from build123d import *

# Parameters (mm, degrees)
SKETCH1_R             = 22.225
BOSS_EXTRUDE1_DEPTH   = 50.8
SKETCH2_R             = 22.225
SKETCH2_R_2           = 15.375
CUT_EXTRUDE1_DEPTH    = 30.1625
SKETCH3_R             = 12.7
CUT_EXTRUDE2_DEPTH    = 49.2125
CUT_EXTRUDE3_START    = -17.4625
SKETCH5_R             = 22.225
SKETCH5_R_2           = 15.875
CUT_EXTRUDE3_DEPTH    = 17.4625
SKETCH6_R             = 8.001
SKETCH6_R_2           = 1.70053
MOTORINTERFACFE_DEPTH = 60.737268518


with BuildPart() as part:
    # Sketch1 → Boss-Extrude1 (new body)
    with BuildSketch(Plane(origin=(0, 0, 0), x_dir=(1, 0, 0), z_dir=(0, 1, 0))):
        with Locations(Location((0, 0, 0), (0, 0, 270))):
            Circle(SKETCH1_R)
    extrude(amount=BOSS_EXTRUDE1_DEPTH)

    # Sketch2 → Cut-Extrude1 (cut)
    with BuildSketch(Plane.XZ):
        with Locations(Location((0, 0, 0), (0, 0, 270))):
            Circle(SKETCH2_R)
        with Locations(Location((0, 0, 0), (0, 0, 270))):
            Circle(SKETCH2_R_2, mode=Mode.SUBTRACT)
    extrude(amount=-CUT_EXTRUDE1_DEPTH, mode=Mode.SUBTRACT)

    # Sketch3 → Cut-Extrude2 (cut)
    with BuildSketch(Plane(origin=(0, 50.8, 0), x_dir=(1, 0, 0), z_dir=(0, 1, 0))):
        with Locations(Location((0, 0, 0), (0, 0, 270))):
            Circle(SKETCH3_R)
    extrude(amount=-CUT_EXTRUDE2_DEPTH, mode=Mode.SUBTRACT)

    # Sketch5 → Cut-Extrude3 (cut)
    with BuildSketch(Plane(origin=(0, 50.8, 0), x_dir=(1, 0, 0), z_dir=(0, 1, 0)).offset(CUT_EXTRUDE3_START)):
        with Locations(Location((0, 0, 0), (0, 0, 90))):
            Circle(SKETCH5_R)
        with Locations(Location((0, 0, 0), (0, 0, 270))):
            Circle(SKETCH5_R_2, mode=Mode.SUBTRACT)
    extrude(amount=CUT_EXTRUDE3_DEPTH, mode=Mode.SUBTRACT)

    # Sketch6 → MotorInterfacfe (cut, through all)
    with BuildSketch(Plane.XZ):
        with Locations(Location((0, 0, 0), (0, 0, 270))):
            Circle(SKETCH6_R)
        with Locations(Location((-7.07105367, 7.07105367, 0), (0, 0, 270))):
            Circle(SKETCH6_R_2)
        with Locations(Location((-7.162899066, -6.970031681, 0), (0, 0, 270))):
            Circle(SKETCH6_R_2)
        with Locations(Location((7.158557907, -7.103864696, 0), (0, 0, 270))):
            Circle(SKETCH6_R_2)
        with Locations(Location((7.036006619, 7.187404798, 0), (0, 0, 270))):
            Circle(SKETCH6_R_2)
    extrude(amount=-MOTORINTERFACFE_DEPTH, mode=Mode.SUBTRACT)


solid = part.part
Work out the finished part from the listing and answer in its coordinate system (mm). A direction names the side the tool comes from. Coordinates: 2 decimals unless noted, no trailing zeros. Loops run counter-clockwise (first coordinate to the right, second up) from the corner with the lowest first, then second, coordinate; pieces in that order, holes last. Notation, with made-up numbers: (82.25, 56) -> (95.25, 56) arc R19 cw to (95.25, 74) -> close; hole circle Ø2 at (9.25, 45.5). An arc over 180 degrees is marked (long way). Answer as CSV lines item,"result".
1) Straight lines are drawn through the part: probe 1 along X at (y, z) = (23, 0) (3 decimals); probe 2 along X at (y, z) = (1.1, 0) (3 decimals); probe 3 along Y at (x, z) = (9, 1). For each, find the intervals that lie inside material, in ascending order.
A:
probe 1,"x = -15.375 to -12.7, 12.7 to 15.375"
probe 2,"x = -15.375 to -8.001, 8.001 to 15.375"
probe 3,"y = 0 to 1.59"
2) For faces 1 (the face through (-15, 30.162, 5)), 2 (the face through (-8.3, 1.587, -0.2)), 3 (the face through (2.403, 0.783, -7.632)), determine the directions among +Z, -Z, +X, -X, +Y, -Y from which every point of the face is accessible in a straight line to the end or side of a thin tool.
A:
face 1,"-Y"
face 2,"+Y"
face 3,"+Y, -Y"
3) The part is cut by section D-D (y = 24.5). Give the vertices of the cut face in (x, z) (3 decimals).
A:
outline,"circle Ø30.75 at (0, 0); hole circle Ø25.4 at (0, 0)"
4) The part is cut by section C-C (z = -6.5). Give the vertices of the cut face in (x, y), and give its area (3 significant figures).
A:
outline,"(-21.25, 30.16) -> (-13.93, 30.16) -> (-13.93, 0) -> (-8.8, 0) -> (-8.8, 1.59) -> (-10.91, 1.59) -> (-10.91, 50.8) -> (-14.48, 50.8) -> (-14.48, 33.34) -> (-21.25, 33.34) -> close; (-5.53, 0) -> (-4.67, 0) -> (-4.67, 1.59) -> (-5.53, 1.59) -> close; (4.67, 0) -> (5.57, 0) -> (5.57, 1.59) -> (4.67, 1.59) -> close; (8.75, 0) -> (13.93, 0) -> (13.93, 30.16) -> (21.25, 30.16) -> (21.25, 33.34) -> (14.48, 33.34) -> (14.48, 50.8) -> (10.91, 50.8) -> (10.91, 1.59) -> (8.75, 1.59) -> close"
area,"382 mm²"
5) For a pull along X with two mould halves and no side action, classify faces 4 (the face through (11, 50.8, -7)), 5 (the face through (-8.73, 0.78, 7.44)), 6 (the face through (-15.497, 41.947, -3.441)) as released by +X, released by -X, zero draft, split by the parting line, or undercut.
A:
face 4,"zero draft"
face 5,"undercut"
face 6,"split by the parting line"
6) The part is cut by section B-B (x = 0). Give the vertices of the cut face in (y, z) (1 decimal).
A:
outline,"(0, -15.4) -> (30.2, -15.4) -> (30.2, -22.2) -> (33.3, -22.2) -> (33.3, -15.9) -> (50.8, -15.9) -> (50.8, -12.7) -> (1.6, -12.7) -> (1.6, -8) -> (0, -8) -> close; (0, 8) -> (1.6, 8) -> (1.6, 12.7) -> (50.8, 12.7) -> (50.8, 15.9) -> (33.3, 15.9) -> (33.3, 22.2) -> (30.2, 22.2) -> (30.2, 15.4) -> (0, 15.4) -> close"
7) The part is cut by section A-A (z = 0). Give the vertices of the cut face in (x, y) (1 decimal), and give its area (3 significant figures).
A:
outline,"(-22.2, 30.2) -> (-15.4, 30.2) -> (-15.4, 0) -> (-8, 0) -> (-8, 1.6) -> (-12.7, 1.6) -> (-12.7, 50.8) -> (-15.9, 50.8) -> (-15.9, 33.3) -> (-22.2, 33.3) -> close; (8, 0) -> (15.4, 0) -> (15.4, 30.2) -> (22.2, 30.2) -> (22.2, 33.3) -> (15.9, 33.3) -> (15.9, 50.8) -> (12.7, 50.8) -> (12.7, 1.6) -> (8, 1.6) -> close"
area,"348 mm²"
8) Flat-ended cylindrical pins translate along their axes: pin 1 (8 mm diameter, centred on x = -5.5, y = 41, fed in from +Z); pin 2 (1 mm diameter, centred on x = -14, y = 15, fed in from -Z); pin 3 (4 mm diameter, centred on x = 7.04, z = 7.19, fed in from +Y); pin 4 (22 mm diameter, centred on x = 4.5, z = 5, fed in from +Y). Find the tip coordinate at first contact, or state that the pin passes through.
A:
pin 1,"stops at z = 15.8"
pin 2,"stops at z = -7.36"
pin 3,"stops at y = 1.59"
pin 4,"stops at y = 50.8"
